from build123d import *

# Parameters (mm, degrees)
SKETCH1_W           = 60
SKETCH1_H           = 120
BOSS_EXTRUDE1_DEPTH = 6.54
SKETCH17_W          = 60
SKETCH17_H          = 40
BOSS_EXTRUDE6_DEPTH = 29
CUT_EXTRUDE1_REACH  = 42
CUT_EXTRUDE2_REACH  = 37.54
SKETCH21_W          = 37.9445377
SKETCH21_H          = 40
SKETCH23_W          = 2
SKETCH23_H          = 36
CUT_EXTRUDE3_DEPTH  = 9
SKETCH24_W          = 2
SKETCH24_H          = 36
CUT_EXTRUDE4_DEPTH  = 9
BOSS_EXTRUDE8_DEPTH = 29
SKETCH36_W          = 60
SKETCH36_H          = 1.8
BOSS_EXTRUDE9_DEPTH = 6.5
FILLET1_R           = 3
FILLET2_R           = 2


with BuildPart() as part:
    # Sketch1 → Boss-Extrude1 (new body)
    with BuildSketch(Plane.XY):
        Rectangle(SKETCH1_W, SKETCH1_H)
    extrude(amount=BOSS_EXTRUDE1_DEPTH)

    # Sketch17 → Boss-Extrude6 (add)
    with BuildSketch(Plane.XY.offset(6.54)):
        with Locations((0, -40)):
            Rectangle(SKETCH17_W, SKETCH17_H)
    extrude(amount=BOSS_EXTRUDE6_DEPTH)

    # Sketch18 → Cut-Extrude1 (cut, up to next)
    with BuildSketch(Plane(origin=(0, -20, 0), x_dir=(1, 0, 0), z_dir=(0, 1, 0)), mode=Mode.PRIVATE) as cut_extrude1_sk1:
        with BuildLine():
            Line((5.334966353, -8.526396136), (21.291300905, -12.825812438))
            add(Edge.make_bspline(
                [(5.334966353, -8.526396136), (-17.854714365, -9.780670981), (-12.49786254, -23.648890313), (-7.141010715, -37.517109645), (13.926544327, -30.768916863), (34.994099369, -24.020724082), (21.291300905, -12.825812438)],
                knots=[1.570796327, 1.570796327, 1.570796327, 3.340987112, 3.340987112, 5.111177898, 5.111177898, 6.881368684, 6.881368684, 6.881368684], degree=2, weights=[1, 0.633215673, 1, 0.633215673, 1, 0.633215673, 1]))
        make_face()
    cut_extrude1_tool1 = extrude(cut_extrude1_sk1.sketch, amount=-CUT_EXTRUDE1_REACH, mode=Mode.PRIVATE) & part.part
    add(cut_extrude1_tool1.solids().sort_by_distance((5.792514, -20, 20.554542))[0], mode=Mode.SUBTRACT)

    # Sketch21 → Cut-Extrude2 (cut, up to next)
    with BuildSketch(Plane.XY.offset(35.54), mode=Mode.PRIVATE) as cut_extrude2_sk1:
        with Locations((5.97226885, -40)):
            Rectangle(SKETCH21_W, SKETCH21_H)
    cut_extrude2_tool1 = extrude(cut_extrude2_sk1.sketch, amount=-CUT_EXTRUDE2_REACH, mode=Mode.PRIVATE) & part.part
    add(cut_extrude2_tool1.solids().sort_by_distance((5.972269, -40, 35.54))[0], mode=Mode.SUBTRACT)

    # Sketch23 → Cut-Extrude3 (cut)
    with BuildSketch(Plane(origin=(-13, 0, 0), x_dir=(0, 0, -1), z_dir=(1, 0, 0))):
        with Locations((-33.04, -40)):
            Rectangle(SKETCH23_W, SKETCH23_H)
    extrude(amount=-CUT_EXTRUDE3_DEPTH, mode=Mode.SUBTRACT)

    # Sketch24 → Cut-Extrude4 (cut)
    with BuildSketch(Plane.ZY.offset(-24.9445377)):
        with Locations((33.04, -40)):
            Rectangle(SKETCH24_W, SKETCH24_H)
    extrude(amount=-CUT_EXTRUDE4_DEPTH, mode=Mode.SUBTRACT)

    # Sketch7 → Boss-Extrude8 (add)
    with BuildSketch(Plane.XY.offset(6.54)):
        with BuildLine():
            Line((-7, 25.533918981), (-18.684094898, 45.817285768))
            ThreePointArc((-18.684094898, 45.817285768), (-20, 46), (-21.294986864, 45.703352481))
            Line((-21.294986864, 45.703352481), (-30, 29.115374119))
            Line((-30, 29.115374119), (-30, 25.533918981))
            Line((-30, 25.533918981), (-7, 25.533918981))
        make_face()
    extrude(amount=BOSS_EXTRUDE8_DEPTH)

    # Sketch36 → Boss-Extrude9 (add)
    with BuildSketch(Plane.XY.offset(6.54)):
        with Locations((0, 54.4)):
            Rectangle(SKETCH36_W, SKETCH36_H)
    extrude(amount=BOSS_EXTRUDE9_DEPTH)

    # Fillet1
    fillet1_edges = [part.edges().sort_by_distance(p)[0] for p in [
        (-7, 25.533918981, 21.04),
    ]]
    fillet(fillet1_edges, radius=FILLET1_R)

    # Fillet2
    fillet2_edges = [part.edges().sort_by_distance(p)[0] for p in [
        (-30, 25.533918981, 21.04),
    ]]
    fillet(fillet2_edges, radius=FILLET2_R)


solid = part.part
Verification items for the finished model (mm, model axes). A direction names the side the tool comes from. Coordinates: 2 decimals unless noted, no trailing zeros. Write each loop counter-clockwise with the first axis right and the second up, starting at its lowest first coordinate (ties: lowest second). Pieces come first, ordered by that corner, then holes. Notation, with made-up numbers: (5.5, 59.25) -> (18.5, 59.25) arc R32 cw to (18.5, 89.25) -> close; hole circle Ø5 at (-16, 28). An arc over 180 degrees is marked (long way). One line per item, written item: value. Start each with the question number.
Q1. Access from +Z, -Z, +X, -X, +Y, -Y to the whole of each face (thin tool, end or side, straight path). Record for faces 5 (the flat face through (0, 53.5, 10)), 6 (the flat face through (-17, -40, 34.04)), 7 (the flat face through (13.201, -39.72, 10.646)), 8 (the cylindrical face through (-9.62, 26.99, 21.24)).
Q2. Mould release check, pull along Y, two halves, no side actions. Record for faces 1 (the flat face through (-17, -40, 32.04)), 2 (the flat face through (27, -40, 32.04)), 3 (the flat face through (-13, -40, 29)), 4 (the flat face through (-7, -60, 10)): pulls with the +Y half, pulls with the -Y half, needs draft (parallel to the pull), parting line crosses it, or undercut.
Q3. Cross-section at A-A on z = 25.5. Enter the section's corners in (x, y), and give its area (3 significant figures).
Q4. Cross-section at B-B on x = 19. Enter the section's corners in (y, z), and give its area (3 significant figures).
Q5. Thickness scan on L1, parallel to Y at x = 13, z = 9.5; L2, parallel to X at y = -23.5, z = 27; L3, parallel to X at y = -47.5, z = 15.5. Record the ranges inside material, lowest first. Write a range as from..to.
Q6. Cross-section at D-D on x = 8. Enter the section's corners in (y, z), and give its area (3 significant figures).
Q7. Cross-section at C-C on y = 18. Enter the section's corners in (x, z).
Q8. Go/stop test with flat-tipped pins: P1, Ø4, axis at x = 27.5, y = -31.5, coming from the -Z side; P2, Ø18, axis at x = 9.5, y = -1, coming from the +Z side; P3, Ø1.6, axis at x = -15.5, z = 33.5, coming from the +Y side; P4, Ø10, axis at x = 15, y = -36, coming from the +Z side. Record where each tip stops, or that it passes through.
Checked values:
1. face 5: +Z, +X, -X
1. face 6: +X
1. face 7: +Z, -Y
1. face 8: +Z, +X
2. face 1: undercut
2. face 2: undercut
2. face 3: needs draft
2. face 4: pulls with the -Y half
3. outline: (-30, -60) -> (-13, -60) -> (-13, -20) -> (-30, -20) -> close; (-30, 27.53) arc R2 ccw to (-28, 25.53) -> (-12.19, 25.53) arc R3 ccw to (-9.59, 30.03) -> (-18.68, 45.82) arc R3.68 ccw to (-21.29, 45.7) -> (-30, 29.12) -> close; (24.94, -60) -> (30, -60) -> (30, -20) -> (24.94, -20) -> close
3. area: 1,150 mm²
4. outline: (-60, 0) -> (60, 0) -> (60, 6.54) -> (55.3, 6.54) -> (55.3, 13.04) -> (53.5, 13.04) -> (53.5, 6.54) -> (-20, 6.54) -> (-20, 12.21) -> (-60, 12.21) -> close
4. area: 1,020 mm²
5. L1: y = -60..-20, 53.5..55.3
5. L2: x = -30..-13, 24.94..30
5. L3: x = -30..-10.93, 23.7..30
6. outline: (-60, 0) -> (60, 0) -> (60, 6.54) -> (55.3, 6.54) -> (55.3, 13.04) -> (53.5, 13.04) -> (53.5, 6.54) -> (-20, 6.54) -> (-20, 9.24) -> (-60, 9.24) -> close
6. area: 905 mm²
7. outline: (-30, 0) -> (30, 0) -> (30, 6.54) -> (-30, 6.54) -> close
8. P1: stops at z = 0
8. P2: stops at z = 6.54
8. P3: stops at y = 41.68
8. P4: stops at z = 12.48
